Could you check a few things on this drawing? It's one solid part, dimensions in mm from its lowest x, y, z. A direction names the side the tool comes from. Coordinates: 2 decimals unless noted, no trailing zeros. Write each loop counter-clockwise with the first axis right and the second up, starting at its lowest first coordinate (ties: lowest second). Pieces come first, ordered by that corner, then holes.
Item 1: Please list where these lines run through material, in increasing order: line 1 (Y direction, x = 6, z = 7.75); line 2 (Z direction, x = 8, y = 10.5); line 3 (X direction, y = 4, z = 2).
Item 2: I want a section at C-C (z = 3.25). Please give me the cut outline in (x, y), and give its area (3 significant figures).
Item 3: I want a section at B-B (z = 5.5). Please give me the cut outline in (x, y), and give its area (3 significant figures).
Item 4: For the marked faces 1, 2, 3, 4 and 5, which set-ups out of +Z, -Z, +X, -X, +Y, -Y let a thin tool reach every point of the face, with its end or its side?
Item 5: I'm going to push flat-ended pins straight in: P1, Ø1, axis at y = 3.5, z = 6, coming from the +X side; P2, Ø1, axis at x = 1.5, z = 4, coming from the +Y side (1 decimal); P3, Ø1.5, axis at x = 10, z = 5.5, coming from the +Y side. Where does each tip first touch, or does it pass through?
Item 6: I want a section at A-A (x = 6.03). Please give me the cut outline in (y, z), and give its area (3 significant figures).
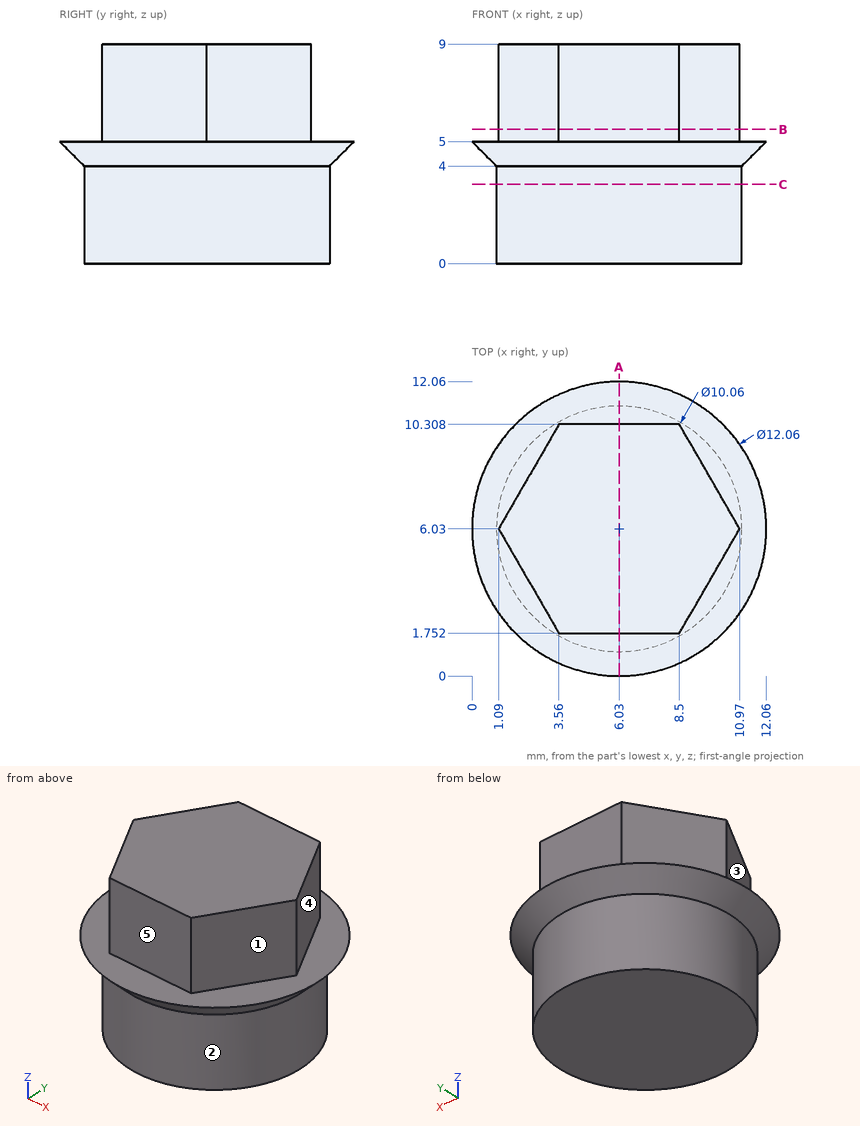
Answer:
1. line 1: y = 1.75 to 10.31
1. line 2: z = 0 to 5
1. line 3: x = 1.43 to 10.63
2. outline: circle Ø10.06 at (6.03, 6.03)
2. area: 79.5 mm2
3. outline: (1.09, 6.03) - (3.56, 1.75) - (8.5, 1.75) - (10.97, 6.03) - (8.5, 10.31) - (3.56, 10.31) - close
3. area: 63.4 mm2
4. face 1: +Z, +X, -Y
4. face 2: -Z
4. face 3: +Z, -X, -Y
4. face 4: +Z, +X, +Y
4. face 5: +Z, +X, -X, -Y
5. P1: stops at x = 9.8
5. P2: stops at y = 9.4
5. P3: stops at y = 11
6. outline: (0, 5) - (1, 4) - (1, 0) - (11.06, 0) - (11.06, 4) - (12.06, 5) - (10.31, 5) - (10.31, 9) - (1.75, 9) - (1.75, 5) - close
6. area: 85.5 mm2
